from build123d import *

# Parameters (mm, degrees)
SKETCH1_R                = 2.5
BOSS_EXTRUDE1_DEPTH      = 15
SKETCH3_R                = 2.5
BOSS_EXTRUDE2_DEPTH      = 7.5
SKETCH4_W                = 5.5
SKETCH4_H                = 5.5
BOSS_EXTRUDE3_DEPTH      = 3
CHAMFER1_SIZE            = 0.5
CHAMFER2_SIZE            = 0.5
CHAMFER3_SIZE            = 0.5
CHAMFER1_OF_MIRROR1_SIZE = 0.5
CHAMFER2_OF_MIRROR1_SIZE = 0.5
SKETCH5_W                = 5.5
SKETCH5_H                = 5.5
BOSS_EXTRUDE4_DEPTH      = 3
CHAMFER4_SIZE            = 0.5
CHAMFER5_SIZE            = 0.5
CHAMFER4_OF_MIRROR2_SIZE = 0.5
CHAMFER5_OF_MIRROR2_SIZE = 0.5


with BuildPart() as part:
    # Sketch1 → Boss-Extrude1 (new body)
    with BuildSketch(Plane.XY):
        Circle(SKETCH1_R)
    extrude(amount=BOSS_EXTRUDE1_DEPTH)

    # Sketch3 → Boss-Extrude2 (add, symmetric)
    with BuildSketch(Plane(origin=(0, 0, 0), x_dir=(1, 0, 0), z_dir=(0, 1, 0))):
        with Locations((0, -7.5)):
            Circle(SKETCH3_R)
    extrude(amount=BOSS_EXTRUDE2_DEPTH, both=True)

    # Sketch4 → Boss-Extrude3 (add)
    with BuildSketch(Plane(origin=(0, 0, 0), x_dir=(-1, 0, 0), z_dir=(0, 0, -1))):
        Rectangle(SKETCH4_W, SKETCH4_H)
    boss_extrude3 = extrude(amount=BOSS_EXTRUDE3_DEPTH)

    # Chamfer1
    chamfer1_edges = [part.edges().sort_by_distance(p)[0] for p in [
        (-2.75, 2.75, -1.5),
    ]]
    chamfer(chamfer1_edges, length=CHAMFER1_SIZE)

    # Chamfer2
    chamfer2_edges = [part.edges().sort_by_distance(p)[0] for p in [
        (2.75, 2.75, -1.5),
        (2.75, -2.75, -1.5),
    ]]
    chamfer(chamfer2_edges, length=CHAMFER2_SIZE)

    # Chamfer3
    chamfer3_edges = [part.edges().sort_by_distance(p)[0] for p in [
        (-2.75, -2.75, -1.5),
    ]]
    chamfer(chamfer3_edges, length=CHAMFER3_SIZE)

    # Mirror1: Boss-Extrude3 across plane
    add(boss_extrude3.mirror(Plane(origin=(0, 0, 7.5), x_dir=(1, 0, 0), z_dir=(0, 0, -1))))

    # Chamfer1 of Mirror1
    chamfer1_of_mirror1_edges = [part.edges().sort_by_distance(p)[0] for p in [
        (-2.75, 2.75, 16.5),
    ]]
    chamfer(chamfer1_of_mirror1_edges, length=CHAMFER1_OF_MIRROR1_SIZE)

    # Chamfer2 of Mirror1
    chamfer2_of_mirror1_edges = [part.edges().sort_by_distance(p)[0] for p in [
        (2.75, 2.75, 16.5),
        (2.75, -2.75, 16.5),
    ]]
    chamfer(chamfer2_of_mirror1_edges, length=CHAMFER2_OF_MIRROR1_SIZE)

    # Sketch5 → Boss-Extrude4 (add)
    with BuildSketch(Plane(origin=(0, 7.5, 0), x_dir=(1, 0, 0), z_dir=(0, 1, 0))):
        with Locations((0, -7.502861602)):
            Rectangle(SKETCH5_W, SKETCH5_H)
    boss_extrude4 = extrude(amount=BOSS_EXTRUDE4_DEPTH)

    # Chamfer4
    chamfer4_edges = [part.edges().sort_by_distance(p)[0] for p in [
        (-2.75, 9, 4.752861602),
        (-2.75, 9, 10.252861602),
        (2.75, 9, 4.752861602),
    ]]
    chamfer(chamfer4_edges, length=CHAMFER4_SIZE)

    # Chamfer5
    chamfer5_edges = [part.edges().sort_by_distance(p)[0] for p in [
        (2.75, 9, 10.252861602),
    ]]
    chamfer(chamfer5_edges, length=CHAMFER5_SIZE)

    # Mirror2: Boss-Extrude4 across plane
    add(boss_extrude4.mirror(Plane(origin=(0, 0, 0), x_dir=(0, 0, 1), z_dir=(0, -1, 0))))

    # Chamfer4 of Mirror2
    chamfer4_of_mirror2_edges = [part.edges().sort_by_distance(p)[0] for p in [
        (-2.75, -9, 4.752861602),
        (-2.75, -9, 10.252861602),
        (2.75, -9, 4.752861602),
    ]]
    chamfer(chamfer4_of_mirror2_edges, length=CHAMFER4_OF_MIRROR2_SIZE)

    # Chamfer5 of Mirror2
    chamfer5_of_mirror2_edges = [part.edges().sort_by_distance(p)[0] for p in [
        (2.75, -9, 10.252861602),
    ]]
    chamfer(chamfer5_of_mirror2_edges, length=CHAMFER5_OF_MIRROR2_SIZE)


solid = part.part
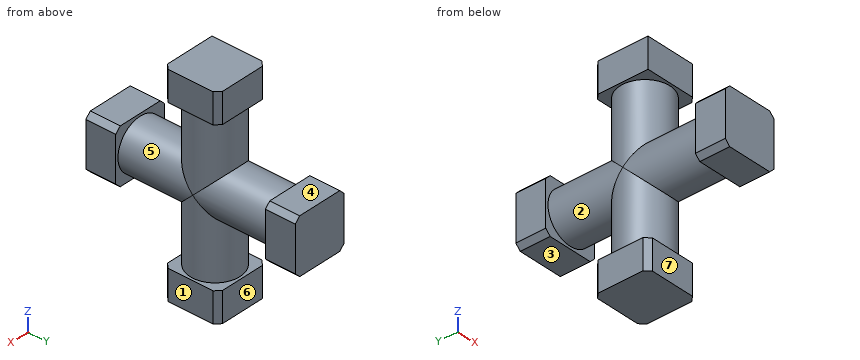
The model under review builds one solid part; all positions refer to its coordinate system, in mm. Face numbers are marked on the shaded views. A direction names the side the tool comes from. Give positions to 0.01 mm unless a question says otherwise; leave off trailing zeros. Order: outer loops, then holes, each group sorted by start corner. A loop starts at its lowest first (then second) coordinate and runs counter-clockwise, first axis right, second up. Notation, with made-up numbers: M 88.25,25.5 L 134.25,25.5 A11 ccw 134.25,37.5 Z; hole C 70.5,-31.75 d2. An arc over 180 degrees is marked long. Answer in a Markdown table with one row per item. Add a question column.
1. Machinability: for the marked faces 4, 5, 6 and 7, which of the approach directions +Z, -Z, +X, -X, +Y, -Y give a long, thin tool a straight path to every point of the face, cutting with its end or side? Answer none if there is none.
2. Mouldability with a two-part tool opening along Z and no side actions: class the marked faces 1, 2 and 3 as released by +Z, released by -Z, zero draft, split by the parting line, or undercut.
3. Add section C-C on y = -8.25. State the section outline as (x, z) points.
4. For pin 1 Ø1.5 at (x, y) = (-1, -8.5) entering from -Z; pin 2 Ø0.9 at (x, y) = (1, -8.5) entering from +Z; pin 3 Ø0.9 at (x, z) = (0.5, 17) entering from +Y, all flat-tipped, find the tip position at first contact; note any pin that passes through.
5. To check wall thickness, follow line 1 along Z through (x, y) = (-1.3, 2.25); line 2 along Y through (x, z) = (0.5, 15.25); line 3 along Z through (x, y) = (-0.8, -2.5). State the ranges of each line that lie inside material, in increasing order.
6. Add section A-A on x = 0. State the section outline as (y, z) points.
7. Add section D-D on x = 1.5. State the section outline as (y, z) points, plus the area to 3 significant figures.
8. Add section B-B on z = 9.5. State the section outline as (x, y) points, plus the area to 3 significant figures.
The answers:
| question | item | result |
|---|---|---|
| 1 | face 4 | +Z, +X, -X, +Y |
| 1 | face 5 | none |
| 1 | face 6 | -Z, +X, -X, +Y |
| 1 | face 7 | -Z, +X, -X, -Y |
| 2 | face 1 | zero draft |
| 2 | face 2 | undercut |
| 2 | face 3 | released by -Z |
| 3 | outline | M -2.75,5.25 L -2.25,4.75 L 2.25,4.75 L 2.75,5.25 L 2.75,9.75 L 2.25,10.25 L -2.25,10.25 L -2.75,9.75 Z |
| 4 | pin 1 | z = 4.75 |
| 4 | pin 2 | z = 10.25 |
| 4 | pin 3 | y = 2.75 |
| 5 | line 1 | -3 to 0, 5.36 to 9.64, 15 to 18 |
| 5 | line 2 | -2.75 to 2.75 |
| 5 | line 3 | -3 to 0, 5.13 to 9.87, 15 to 18 |
| 6 | outline | M -10.5,4.75 L -7.5,4.75 L -7.5,5 L -2.5,5 L -2.5,0 L -2.75,0 L -2.75,-3 L 2.75,-3 L 2.75,0 L 2.5,0 L 2.5,5 L 7.5,5 L 7.5,4.75 L 10.5,4.75 L 10.5,10.25 L 7.5,10.25 L 7.5,10 L 2.5,10 L 2.5,15 L 2.75,15 L 2.75,18 L -2.75,18 L -2.75,15 L -2.5,15 L -2.5,10 L -7.5,10 L -7.5,10.25 L -10.5,10.25 Z |
| 7 | outline | M -10.5,4.75 L -7.5,4.75 L -7.5,5.5 L -2,5.5 L -2,0 L -2.75,0 L -2.75,-3 L 2.75,-3 L 2.75,0 L 2,0 L 2,5.5 L 7.5,5.5 L 7.5,4.75 L 10.5,4.75 L 10.5,10.25 L 7.5,10.25 L 7.5,9.5 L 2,9.5 L 2,15 L 2.75,15 L 2.75,18 L -2.75,18 L -2.75,15 L -2,15 L -2,9.5 L -7.5,9.5 L -7.5,10.25 L -10.5,10.25 Z |
| 7 | area | 170 mm2 |
| 8 | outline | M -2.75,-10.5 L 2.75,-10.5 L 2.75,-7.5 L 1.5,-7.5 L 1.5,-2 A2.5 ccw 1.5,2 L 1.5,7.5 L 2.75,7.5 L 2.75,10.5 L -2.75,10.5 L -2.75,7.5 L -1.5,7.5 L -1.5,2 A2.5 ccw -1.5,-2 L -1.5,-7.5 L -2.75,-7.5 Z |
| 8 | area | 83.6 mm2 |
